```python
from build123d import *

# Parameters (mm, degrees)
BOSS_EXTRUDE1_DEPTH = 19.05
FILLET1_R           = 1.27
SKETCH3_W           = 2.286
SKETCH3_H           = 4.572
BOSS_EXTRUDE2_DEPTH = 19.05
SKETCH4_W           = 11.43
SKETCH4_H           = 3.302
CUT_EXTRUDE2_DEPTH  = 3.286


with BuildPart() as part:
    # Sketch2 → Boss-Extrude1 (new body)
    with BuildSketch(Plane.XY):
        Polygon((-50.411, 53.12524277), (-50.411, 61.17475723), (-48.125, 59.90475723), (-48.125, 62.192675039), (-52.411, 64.57378615), (-52.411, 49.72621385), (-48.125, 52.107324961), (-48.125, 54.39524277), align=None)
    extrude(amount=BOSS_EXTRUDE1_DEPTH)

    # Fillet1
    fillet1_edges = [part.edges().sort_by_distance(p)[0] for p in [
        (-52.411, 49.72621385, 9.525),
        (-52.411, 64.57378615, 9.525),
    ]]
    fillet(fillet1_edges, radius=FILLET1_R)

    # Sketch3 → Boss-Extrude2 (add, through all)
    with BuildSketch(Plane.XY.offset(19.05)):
        with Locations((-49.268, 49.821324961)):
            Rectangle(SKETCH3_W, SKETCH3_H)
    extrude(amount=-BOSS_EXTRUDE2_DEPTH)

    # Sketch4 → Cut-Extrude2 (cut, through all)
    with BuildSketch(Plane.ZY.offset(50.411)):
        with Locations((9.525, 49.186324961)):
            Rectangle(SKETCH4_W, SKETCH4_H)
    extrude(amount=-CUT_EXTRUDE2_DEPTH, mode=Mode.SUBTRACT)


solid = part.part
```
Check sheet for the modelled part. Datum: model origin and axes. Units: mm. A direction names the side the tool comes from. Coordinates: 2 decimals unless noted, no trailing zeros. Write each loop counter-clockwise with the first axis right and the second up, starting at its lowest first coordinate (ties: lowest second). Pieces come first, ordered by that corner, then holes. Notation, with made-up numbers: M -13.75,-29.75 L 42.25,-29.75 A27 ccw 42.25,1.25 Z; hole C 37,-7 d2. An arc over 180 degrees is marked long. Write item = value, one per line. Start each with the question number.
1. Sectioned sample at A-A (x = -48.8). Record the cut outline in (y, z).
2. Go/stop test with flat-tipped pins: pin 1 (1 mm diameter, centred on y = 50, z = 17, fed in from -X); pin 2 (1.1 mm diameter, centred on x = -49, z = 11.5, fed in from -Y); pin 3 (2 mm diameter, centred on x = -52, z = 5.5, fed in from -Y). Record where each tip stops, or that it passes through.
3. Mould release check, pull along Z, two halves, no side actions. Record for faces 3 (the flat face through (-51, 56, 0)), 4 (the flat face through (-49, 50.837, 9)), 5 (the flat face through (-50.411, 49, 17)): pulls with the +Z half, pulls with the -Z half, needs draft (parallel to the pull), parting line crosses it, or undercut.
4. Sectioned sample at D-D (z = 7.75). Record the cut outline in (x, y) (3 decimals).
5. Sectioned sample at B-B (z = 18). Record the cut outline in (x, y) (3 decimals).
6. Tool access check on faces 1 (the flat face through (-49.31, 62.85, 9.39)), 2 (the flat face through (-49.25, 53.77, 9.39)). Record the directions out of +Z, -Z, +X, -X, +Y, -Y that give a thin tool (end or side, any length) a straight path to the whole face; none if there is none.
7. Thickness scan on probe 1 along Z at (x, y) = (-49.15, 48.5); probe 2 along Y at (x, z) = (-49.7, 16); probe 3 along Y at (x, z) = (-48.75, 13.25). Record the ranges inside material, lowest first.
8. Sectioned sample at C-C (y = 56.25). Record the cut outline in (x, z), then the cut area to 3 significant figures.
The answers:
q1.outline = M 47.54,0 L 54.02,0 L 54.02,19.05 L 47.54,19.05 L 47.54,15.24 L 50.84,15.24 L 50.84,3.81 L 47.54,3.81 Z; M 60.28,0 L 62.57,0 L 62.57,19.05 L 60.28,19.05 Z
q2.pin_1 = -50.41
q2.pin_2 = 50.84
q2.pin_3 = 50.61
q3.face_3 = pulls with the -Z half
q3.face_4 = undercut
q3.face_5 = needs draft
q4.outline = M -52.411,51.885 A1.27 ccw -50.524,50.774 L -50.411,50.837 L -48.125,50.837 L -48.125,54.395 L -50.411,53.125 L -50.411,61.175 L -48.125,59.905 L -48.125,62.193 L -50.524,63.526 A1.27 ccw -52.411,62.415 Z
q5.outline = M -52.411,51.885 A1.27 ccw -50.524,50.774 L -50.411,50.837 L -50.411,47.535 L -48.125,47.535 L -48.125,54.395 L -50.411,53.125 L -50.411,61.175 L -48.125,59.905 L -48.125,62.193 L -50.524,63.526 A1.27 ccw -52.411,62.415 Z
q6.face_1 = +Z, -Z, +X, +Y
q6.face_2 = +Z, -Z
q7.probe_1 = 0 to 3.81, 15.24 to 19.05
q7.probe_2 = 47.54 to 53.52, 60.78 to 63.07
q7.probe_3 = 50.84 to 54.05, 60.25 to 62.54
q8.outline = M -52.41,0 L -50.41,0 L -50.41,19.05 L -52.41,19.05 Z
q8.area = 38.1 mm²
